from build123d import *

# Parameters (mm, degrees)
BOSS_EXTRUDE2_DEPTH = 10
BOSS_EXTRUDE3_START = 8
BOSS_EXTRUDE3_DEPTH = 8
CUT_EXTRUDE1_REACH  = 23.149
SKETCH3_R           = 1.75
BOSS_EXTRUDE4_DEPTH = 3.204301934
FILLET2_R           = 8


with BuildPart() as part:
    # Sketch1 → Boss-Extrude2 (new body)
    with BuildSketch(Plane.XY):
        with BuildLine():
            Line((2.115260933, -1.332543126), (-1.082842756, -6.409169335))
            ThreePointArc((-1.082842756, -6.409169335), (5.499678326, -3.464612288), (5.313364545, 3.744082959))
            Line((5.313364545, 3.744082959), (2.115260933, -1.332543126))
        make_face()
        with BuildLine():
            Line((-3.447804083, -0.782717707), (-5.313364545, -3.744082959))
            ThreePointArc((-5.313364545, -3.744082959), (-3.464612288, -5.499678326), (-1.082842756, -6.409169335))
            Line((-1.082842756, -6.409169335), (2.115260933, -1.332543126))
            ThreePointArc((2.115260933, -1.332543126), (0.553465034, -2.437965639), (-1.332543188, -2.115260895))
            Line((-1.332543188, -2.115260895), (-3.447804083, -0.782717707))
        make_face()
        with BuildLine():
            Line((-5.313364545, -3.744082959), (-9.577502747, -10.512917822))
            Line((-9.577502747, -10.512917822), (-5.346980957, -13.178004198))
            Line((-5.346980957, -13.178004198), (-1.082842756, -6.409169335))
            ThreePointArc((-1.082842756, -6.409169335), (-3.464612288, -5.499678326), (-5.313364545, -3.744082959))
        make_face()
        with BuildLine():
            ThreePointArc((2.5, 0), (2.401890124, -0.693486722), (2.115260933, -1.332543126))
            Line((2.115260933, -1.332543126), (5.313364545, 3.744082959))
            ThreePointArc((5.313364545, 3.744082959), (3.464612288, 5.499678326), (1.082842756, 6.409169335))
            Line((1.082842756, 6.409169335), (-0.782717707, 3.447804083))
            Line((-0.782717707, 3.447804083), (1.332543188, 2.115260895))
            ThreePointArc((1.332543188, 2.115260895), (2.188761975, 1.208023599), (2.5, 0))
        make_face()
        with BuildLine():
            ThreePointArc((1.082842756, 6.409169335), (3.464612288, 5.499678326), (5.313364545, 3.744082959))
            Line((5.313364545, 3.744082959), (9.577502747, 10.512917822))
            Line((9.577502747, 10.512917822), (5.346980957, 13.178004198))
            Line((5.346980957, 13.178004198), (1.082842756, 6.409169335))
        make_face()
    extrude(amount=-BOSS_EXTRUDE2_DEPTH)

    # Sketch2 → Boss-Extrude3 (add)
    with BuildSketch(Plane.XY.offset(BOSS_EXTRUDE3_START)):
        with BuildLine():
            Line((5.313364545, 3.744082959), (9.577502747, 10.512917822))
            Line((9.577502747, 10.512917822), (5.346980957, 13.178004198))
            Line((5.346980957, 13.178004198), (-0.782717707, 3.447804083))
            Line((-0.782717707, 3.447804083), (1.332543188, 2.115260895))
            ThreePointArc((1.332543188, 2.115260895), (2.115260895, -1.332543188), (-1.332543188, -2.115260895))
            Line((-1.332543188, -2.115260895), (-3.447804083, -0.782717707))
            Line((-3.447804083, -0.782717707), (-9.577502747, -10.512917822))
            Line((-9.577502747, -10.512917822), (-5.346980957, -13.178004198))
            Line((-5.346980957, -13.178004198), (-1.082842756, -6.409169335))
            ThreePointArc((-1.082842756, -6.409169335), (5.499678326, -3.464612288), (5.313364545, 3.744082959))
        make_face()
    extrude(amount=-BOSS_EXTRUDE3_DEPTH)

    # Sketch3 → Cut-Extrude1 (cut, up to next)
    with BuildSketch(Plane(origin=(2.115260895, -1.332543188, 0), x_dir=(0, 0, -1), z_dir=(0.8461043578704048, -0.5330172751353468, 0)), mode=Mode.PRIVATE) as cut_extrude1_sk1:
        with Locations(Location((1.124998711, 8, 0), (0, 0, 90))):
            Circle(SKETCH3_R)
    cut_extrude1_tool1 = extrude(cut_extrude1_sk1.sketch, amount=-CUT_EXTRUDE1_REACH, mode=Mode.PRIVATE) & part.part
    # Sketch3 → Cut-Extrude1 (cut, up to next)
    with BuildSketch(Plane(origin=(2.115260895, -1.332543188, 0), x_dir=(0, 0, -1), z_dir=(0.8461043578704048, -0.5330172751353468, 0)), mode=Mode.PRIVATE) as cut_extrude1_sk2:
        with Locations(Location((1.124998711, -8, 0), (0, 0, 90))):
            Circle(SKETCH3_R)
    cut_extrude1_tool2 = extrude(cut_extrude1_sk2.sketch, amount=-CUT_EXTRUDE1_REACH, mode=Mode.PRIVATE) & part.part
    add(cut_extrude1_tool1.solids().sort_by_distance((6.379399, 5.436292, -1.124999))[0], mode=Mode.SUBTRACT)
    add(cut_extrude1_tool2.solids().sort_by_distance((-2.148877, -8.101378, -1.124999))[0], mode=Mode.SUBTRACT)

    # Sketch4 → Boss-Extrude4 (add)
    with BuildSketch(Plane(origin=(0, 0, -10), x_dir=(-1, 0, 0), z_dir=(0, 0, -1))):
        with BuildLine():
            Line((1.082842756, -6.409169335), (5.346980957, -13.178004198))
            Line((5.346980957, -13.178004198), (9.577502747, -10.512917822))
            Line((9.577502747, -10.512917822), (3.447804083, -0.782717707))
            Line((3.447804083, -0.782717707), (1.332543188, -2.115260895))
            ThreePointArc((1.332543188, -2.115260895), (-2.115260895, -1.332543188), (-1.332543188, 2.115260895))
            Line((-1.332543188, 2.115260895), (0.782717707, 3.447804083))
            Line((0.782717707, 3.447804083), (-5.346980957, 13.178004198))
            Line((-5.346980957, 13.178004198), (-9.577502747, 10.512917822))
            Line((-9.577502747, 10.512917822), (-5.313364545, 3.744082959))
            ThreePointArc((-5.313364545, 3.744082959), (-5.499678326, -3.464612288), (1.082842756, -6.409169335))
        make_face()
    extrude(amount=BOSS_EXTRUDE4_DEPTH)

    # Fillet2
    fillet2_edges = [part.edges().sort_by_distance(p)[0] for p in [
        (-7.462241852, -11.84546101, -13.204301934),
        (-7.462241852, -11.84546101, 8),
        (7.462241852, 11.84546101, 8),
        (7.462241852, 11.84546101, -13.204301934),
    ]]
    fillet(fillet2_edges, radius=FILLET2_R)


solid = part.part
Work out the finished part from the listing and answer in its coordinate system (mm). A direction names the side the tool comes from. Round coordinates to 2 decimals unless told otherwise and drop trailing zeros. Write each loop counter-clockwise with the first axis right and the second up, starting at its lowest first coordinate (ties: lowest second). Pieces come first, ordered by that corner, then holes.
1) Straight lines are drawn through the part: line 1 (Y direction, x = 0.25, z = -0.5); line 2 (Z direction, x = 5, y = 5.25); line 3 (Y direction, x = 1.75, z = -0.25). For each, find the intervals that lie inside material, in ascending order.
2) A cutting plane is placed at A-A (x = 0). Give the vertices of the cut face in (y, z), plus the area to 3 significant figures.
3) Given pin 1 Ø6 at (x, z) = (-1, -10) entering from +Y; pin 2 Ø4 at (y, z) = (-8, -8.5) entering from -X; pin 3 Ø8 at (x, z) = (6.5, 4) entering from +Y, each flat-ended and moving along its own axis, determine where each tip first touches the part or whether it passes through.
4) A tool of negligible diameter and unlimited length cuts with its end or side. For faces 1 (the flat face through (0.29, 2.77, -2.45)), 2 (the flat face through (-7.433, -11.864, -2.566)), 3 (the flat face through (7.48, 7.18, -2.45)), from which of +Z, -Z, +X, -X, +Y, -Y can it reach the whole face along a straight path? Write none if from no direction.
5) The mould has two halves that part along X. Classify faces 4 (the flat face through (-2.405, -1.44, -2.454)), 5 (the cylindrical face through (-6.15, -9.83, 5.72)), 6 (the flat face through (2, -3, -13.204)): pulls with the +X half, pulls with the -X half, needs draft (parallel to the pull), parting line crosses it, or undercut.
6) A cutting plane is placed at B-B (z = -11). Give the vertices of the cut face in (x, y).
7) A cutting plane is placed at C-C (z = 5.25). Give the vertices of the cut face in (x, y), plus the area to 3 significant figures.
Completed:
1. line 1: y = -6.5 to -2.49, 2.8 to 5.09
1. line 2: z = -13.13 to -2.63, 0.38 to 7.92
1. line 3: y = -6.26 to -1.79, 1.79 to 6.56
2. outline: (-6.5, -13.2) - (-2.5, -13.2) - (-2.5, 8) - (-6.5, 8) - close; (2.95, -13.2) - (4.69, -13.2) - (4.69, 8) - (2.95, 8) - close
2. area: 122 mm2
3. pin 1: stops at y = 7.87
3. pin 2: stops at x = -9.25
3. pin 3: stops at y = 13.18
4. face 1: +Z, -Z, -X
4. face 2: +Z, -Z, -X, -Y
4. face 3: +Z, -Z, +X
5. face 4: undercut
5. face 5: pulls with the -X half
5. face 6: needs draft
6. outline: (-8.25, -8.41) - (-4.02, -11.08) - (-1.08, -6.41) arc R6.5 ccw to (5.31, 3.74) - (8.25, 8.41) - (4.02, 11.08) - (-0.78, 3.45) - (1.33, 2.12) arc R2.5 cw to (-1.33, -2.12) - (-3.45, -0.78) - close
7. outline: (-8.53, -8.85) - (-4.3, -11.52) - (-1.08, -6.41) arc R6.5 ccw to (5.31, 3.74) - (8.53, 8.85) - (4.3, 11.52) - (-0.78, 3.45) - (1.33, 2.12) arc R2.5 cw to (-1.33, -2.12) - (-3.45, -0.78) - close
7. area: 133 mm2
